The listing builds one solid part. Answer for the finished solid, in the listing's coordinates (mm). Face numbers are marked on the shaded views. A direction names the side the tool comes from. Round coordinates to 2 decimals unless told otherwise and drop trailing zeros. Order: outer loops, then holes, each group sorted by start corner. A loop starts at its lowest first (then second) coordinate and runs counter-clockwise, first axis right, second up. Notation, with made-up numbers: (-38, -1.5) -> (17, -1.5) arc R26 cw to (17, 21.5) -> close; hole circle Ø1 at (-0.5, -27). An arc over 180 degrees is marked (long way). Return JSON: item names as keys, results as strings. Group by question number.
(1) The part is cut by section B-B (x = 23.9). Determine the outline of the cut face in (y, z).
(2) The part is cut by section A-A (z = 18.5). Determine the outline of the cut face in (x, y), plus the area to 3 significant figures.
(3) Consider line 1 (Y direction, x = 0, z = 5.25); line 2 (X direction, y = -35, z = 2.75); line 3 (Y direction, x = 8, z = 14). Determine where each line is inside the solid, lowest interval first. Write a range as [from, to].
(4) The part is cut by section C-C (y = 42.5). Determine the outline of the cut face in (x, z), plus the area to 3 significant figures.
(5) Which of the six approach directions +Z, -Z, +X, -X, +Y, -Y give full straight-line access (tool end or side, diameter ignored) to the marked faces 1, 2, 3, 4 and 5?
(6) The part is cut by section D-D (x = 0). Count the separate pieces of the cut face and the enclosed holes in it, plus the area to 3 significant figures.
(7) Each of these flat-tipped pins is pushed along its axis until it touches: pin 1 (1.1 mm diameter, centred on x = -37.5, y = -14.5, fed in from -Z); pin 2 (2.5 mm diameter, centred on x = 37.5, z = 10, fed in from +Y); pin 3 (4 mm diameter, centred on y = -24, z = 7.5, fed in from +X); pin 4 (2 mm diameter, centred on x = -37, y = 13.5, fed in from +Z). Where does it stop, or does it pass through?
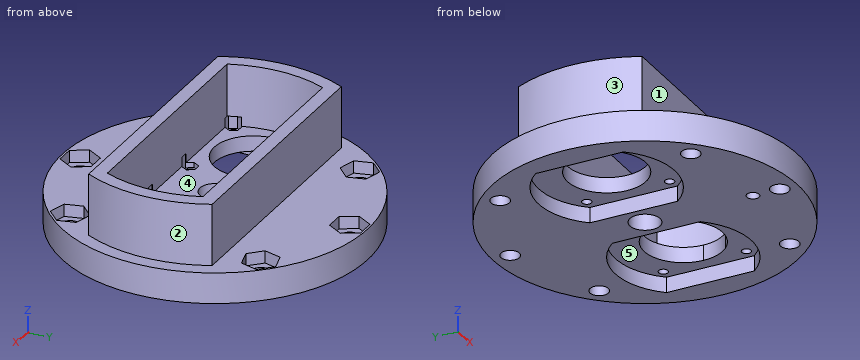
from build123d import *

# Parameters (mm, degrees)
SKETCH2_R               = 49.5
BOSS_EXTRUDE1_DEPTH     = 10
SKETCH1_R               = 1.5
SKETCH1_R_2             = 12.7
CUT_EXTRUDE1_DEPTH      = 5
SKETCH1_12_R            = 4.9
SKETCH1_12_R_2          = 2
CUT_EXTRUDE2_DEPTH      = 45
SKETCH1_13_R            = 1.5
CUT_EXTRUDE3_DEPTH      = 10
BOSS_EXTRUDE2_DEPTH     = 20
SKETCH5_R               = 3
CUT_EXTRUDE4_DEPTH      = 20
SKETCH6_R               = 3
CUT_EXTRUDE5_DEPTH      = 4
CUT_EXTRUDE6_DEPTH      = 3
CUT_EXTRUDE6_DEPTH_BACK = 1.65


with BuildPart() as part:
    # Sketch2 → Boss-Extrude1 (new body)
    with BuildSketch(Plane.XY):
        Circle(SKETCH2_R)
    extrude(amount=BOSS_EXTRUDE1_DEPTH)

    # Sketch1 → Cut-Extrude1 (cut)
    # profile 1 of 2: a face of its own
    with BuildSketch(Plane(origin=(0, 0, 0), x_dir=(-1, 0, 0), z_dir=(0, 0, 1))):
        with BuildLine():
            Line((-7, 14.240786495), (-7, -14.240786495))
            ThreePointArc((-7, -14.240786495), (-23.9, -22.1), (-40.8, -14.240786495))
            Line((-40.8, -14.240786495), (-40.8, 14.240786495))
            ThreePointArc((-40.8, 14.240786495), (-23.9, 22.1), (-7, 14.240786495))
        make_face()
        with Locations(Location((-37.370384182, 13.470384182, 0), (0, 0, 180))):
            Circle(SKETCH1_R, mode=Mode.SUBTRACT)
        with Locations(Location((-10.464971157, 13.435028843, 0), (0, 0, 180))):
            Circle(SKETCH1_R, mode=Mode.SUBTRACT)
        with Locations(Location((-10.464971157, -13.435028843, 0), (0, 0, 180))):
            Circle(SKETCH1_R, mode=Mode.SUBTRACT)
        with Locations(Location((-37.370384182, -13.470384182, 0), (0, 0, 180))):
            Circle(SKETCH1_R, mode=Mode.SUBTRACT)
        with Locations(Location((-23.9, 0, 0), (0, 0, 180))):
            Circle(SKETCH1_R_2, mode=Mode.SUBTRACT)
    # profile 2 of 2: a face of its own
    with BuildSketch(Plane(origin=(0, 0, 0), x_dir=(-1, 0, 0), z_dir=(0, 0, 1))):
        with BuildLine():
            Line((7, 14.240786495), (7, -14.240786495))
            ThreePointArc((7, -14.240786495), (23.9, -22.1), (40.8, -14.240786495))
            Line((40.8, -14.240786495), (40.8, 14.240786495))
            ThreePointArc((40.8, 14.240786495), (23.9, 22.1), (7, 14.240786495))
        make_face()
        with Locations(Location((10.464971157, 13.435028843, 0), (0, 0, 180))):
            Circle(SKETCH1_R, mode=Mode.SUBTRACT)
        with Locations(Location((10.464971157, -13.435028843, 0), (0, 0, 180))):
            Circle(SKETCH1_R, mode=Mode.SUBTRACT)
        with Locations(Location((37.370384182, -13.470384182, 0), (0, 0, 180))):
            Circle(SKETCH1_R, mode=Mode.SUBTRACT)
        with Locations(Location((37.370384182, 13.470384182, 0), (0, 0, 180))):
            Circle(SKETCH1_R, mode=Mode.SUBTRACT)
        with Locations(Location((23.9, 0, 0), (0, 0, 180))):
            Circle(SKETCH1_R_2, mode=Mode.SUBTRACT)
    extrude(amount=CUT_EXTRUDE1_DEPTH, mode=Mode.SUBTRACT)

    # Sketch1<12> → Cut-Extrude2 (cut)
    with BuildSketch(Plane(origin=(0, 0, 0), x_dir=(-1, 0, 0), z_dir=(0, 0, 1))):
        Circle(SKETCH1_12_R)
        with Locations((0, 35)):
            Circle(SKETCH1_12_R_2)
        with BuildLine():
            Line((-11.2, 0), (-23.9, 0))
            Line((-23.9, 0), (-36.6, 0))
            ThreePointArc((-36.6, 0), (-23.9, -12.7), (-11.2, 0))
        make_face()
        with BuildLine():
            Line((-14.919743879, 8.980256121), (-23.9, 0))
            Line((-23.9, 0), (-11.2, 0))
            ThreePointArc((-11.2, 0), (-12.166729937, 4.860079591), (-14.919743879, 8.980256121))
        make_face()
        with BuildLine():
            Line((-32.880256121, 8.980256121), (-23.9, 0))
            Line((-23.9, 0), (-14.919743879, 8.980256121))
            ThreePointArc((-14.919743879, 8.980256121), (-23.9, 12.7), (-32.880256121, 8.980256121))
        make_face()
        with BuildLine():
            Line((-36.6, 0), (-23.9, 0))
            Line((-23.9, 0), (-32.880256121, 8.980256121))
            ThreePointArc((-32.880256121, 8.980256121), (-35.633270063, 4.860079591), (-36.6, 0))
        make_face()
        with BuildLine():
            Line((11.2, 0), (23.9, 0))
            Line((23.9, 0), (36.6, 0))
            ThreePointArc((36.6, 0), (23.9, 12.7), (11.2, 0))
        make_face()
        with BuildLine():
            Line((36.6, 0), (23.9, 0))
            Line((23.9, 0), (11.2, 0))
            ThreePointArc((11.2, 0), (23.9, -12.7), (36.6, 0))
        make_face()
    extrude(amount=CUT_EXTRUDE2_DEPTH, mode=Mode.SUBTRACT)

    # Sketch1<13> → Cut-Extrude3 (cut)
    with BuildSketch(Plane(origin=(0, 0, 0), x_dir=(-1, 0, 0), z_dir=(0, 0, 1))):
        with Locations(Location((-37.370384182, 13.470384182, 0), (0, 0, 180))):
            Circle(SKETCH1_13_R)
        with Locations(Location((-10.464971157, 13.435028843, 0), (0, 0, 180))):
            Circle(SKETCH1_13_R)
        with Locations(Location((-10.464971157, -13.435028843, 0), (0, 0, 180))):
            Circle(SKETCH1_13_R)
        with Locations(Location((-37.370384182, -13.470384182, 0), (0, 0, 180))):
            Circle(SKETCH1_13_R)
        with Locations(Location((10.464971157, 13.435028843, 0), (0, 0, 180))):
            Circle(SKETCH1_13_R)
        with Locations(Location((10.464971157, -13.435028843, 0), (0, 0, 180))):
            Circle(SKETCH1_13_R)
        with Locations(Location((37.370384182, -13.470384182, 0), (0, 0, 180))):
            Circle(SKETCH1_13_R)
        with Locations(Location((37.370384182, 13.470384182, 0), (0, 0, 180))):
            Circle(SKETCH1_13_R)
    extrude(amount=CUT_EXTRUDE3_DEPTH, mode=Mode.SUBTRACT)

    # Sketch4 → Boss-Extrude2 (add)
    with BuildSketch(Plane.XY.offset(10)):
        with BuildLine():
            Line((-40.311288741, -20), (40.311288741, -20))
            ThreePointArc((40.311288741, -20), (45, 0), (40.311288741, 20))
            Line((40.311288741, 20), (-40.311288741, 20))
            ThreePointArc((-40.311288741, 20), (-45, 0), (-40.311288741, -20))
        make_face()
        with BuildLine():
            Line((37.416573868, -15.5), (-37.416573868, -15.5))
            ThreePointArc((-37.416573868, -15.5), (-40.5, 0), (-37.416573868, 15.5))
            Line((-37.416573868, 15.5), (37.416573868, 15.5))
            ThreePointArc((37.416573868, 15.5), (40.5, 0), (37.416573868, -15.5))
        make_face(mode=Mode.SUBTRACT)
    extrude(amount=BOSS_EXTRUDE2_DEPTH)

    # Sketch5 → Cut-Extrude4 (cut)
    with BuildSketch(Plane.XY.offset(10)):
        with Locations((0, 43.7)):
            Circle(SKETCH5_R)
        with Locations((30.900566338, 30.900566338)):
            Circle(SKETCH5_R)
        with Locations((30.900566338, -30.900566338)):
            Circle(SKETCH5_R)
        with Locations((0, -43.7)):
            Circle(SKETCH5_R)
        with Locations((-30.900566338, -30.900566338)):
            Circle(SKETCH5_R)
        with Locations((-30.900566338, 30.900566338)):
            Circle(SKETCH5_R)
    extrude(amount=-CUT_EXTRUDE4_DEPTH, mode=Mode.SUBTRACT)

    # Sketch6 → Cut-Extrude5 (cut)
    # profile 1 of 6: a face of its own
    with BuildSketch(Plane.XY.offset(10)):
        Polygon((-2.915618859, 38.65), (2.915618859, 38.65), (5.831237719, 43.7), (2.915618859, 48.75), (-2.915618859, 48.75), (-5.831237719, 43.7), align=None)
        with Locations((0, 43.7)):
            Circle(SKETCH6_R, mode=Mode.SUBTRACT)
    # profile 2 of 6: a face of its own
    with BuildSketch(Plane.XY.offset(10)):
        Polygon((25.268023226, 29.39133096), (29.39133096, 25.268023226), (35.023874072, 26.777258604), (36.53310945, 32.409801716), (32.409801716, 36.53310945), (26.777258604, 35.023874072), align=None)
        with Locations((30.900566338, 30.900566338)):
            Circle(SKETCH6_R, mode=Mode.SUBTRACT)
    # profile 3 of 6: a face of its own
    with BuildSketch(Plane.XY.offset(10)):
        Polygon((29.39133096, -25.268023226), (25.268023226, -29.39133096), (26.777258604, -35.023874072), (32.409801716, -36.53310945), (36.53310945, -32.409801716), (35.023874072, -26.777258604), align=None)
        with Locations((30.900566338, -30.900566338)):
            Circle(SKETCH6_R, mode=Mode.SUBTRACT)
    # profile 4 of 6: a face of its own
    with BuildSketch(Plane.XY.offset(10)):
        Polygon((2.915618859, -38.65), (-2.915618859, -38.65), (-5.831237719, -43.7), (-2.915618859, -48.75), (2.915618859, -48.75), (5.831237719, -43.7), align=None)
        with Locations((0, -43.7)):
            Circle(SKETCH6_R, mode=Mode.SUBTRACT)
    # profile 5 of 6: a face of its own
    with BuildSketch(Plane.XY.offset(10)):
        Polygon((-25.268023226, -29.39133096), (-29.39133096, -25.268023226), (-35.023874072, -26.777258604), (-36.53310945, -32.409801716), (-32.409801716, -36.53310945), (-26.777258604, -35.023874072), align=None)
        with Locations((-30.900566338, -30.900566338)):
            Circle(SKETCH6_R, mode=Mode.SUBTRACT)
    # profile 6 of 6: a face of its own
    with BuildSketch(Plane.XY.offset(10)):
        Polygon((-26.777258604, 35.023874072), (-32.409801716, 36.53310945), (-36.53310945, 32.409801716), (-35.023874072, 26.777258604), (-29.39133096, 25.268023226), (-25.268023226, 29.39133096), align=None)
    extrude(amount=-CUT_EXTRUDE5_DEPTH, mode=Mode.SUBTRACT)

    # Sketch7 → Cut-Extrude6 (cut, two sides: drawn at the far end of the back side and taken through both)
    with BuildSketch(Plane.XY.offset(10).offset(-CUT_EXTRUDE6_DEPTH_BACK)):
        Polygon((-34.887778024, 13.470384182), (-36.129081103, 15.620384182), (-38.61168726, 15.620384182), (-39.852990339, 13.470384182), (-38.61168726, 11.320384182), (-36.129081103, 11.320384182), align=None)
        Polygon((-9.18831274, -11.320384182), (-11.670918897, -11.320384182), (-12.912221976, -13.470384182), (-11.670918897, -15.620384182), (-9.18831274, -15.620384182), (-7.947009661, -13.470384182), align=None)
        Polygon((-36.129081103, -11.320384182), (-34.887778024, -13.470384182), (-36.129081103, -15.620384182), (-38.61168726, -15.620384182), (-39.852990339, -13.470384182), (-38.61168726, -11.320384182), align=None)
        Polygon((36.129081103, 11.320384182), (34.887778024, 13.470384182), (36.129081103, 15.620384182), (38.61168726, 15.620384182), (39.852990339, 13.470384182), (38.61168726, 11.320384182), align=None)
        Polygon((9.18831274, 11.320384182), (11.670918897, 11.320384182), (12.912221976, 13.470384182), (11.670918897, 15.620384182), (9.18831274, 15.620384182), (7.947009661, 13.470384182), align=None)
        Polygon((7.947009661, -13.470384182), (9.18831274, -11.320384182), (11.670918897, -11.320384182), (12.912221976, -13.470384182), (11.670918897, -15.620384182), (9.18831274, -15.620384182), align=None)
        Polygon((38.61168726, -11.320384182), (36.129081103, -11.320384182), (34.887778024, -13.470384182), (36.129081103, -15.620384182), (38.61168726, -15.620384182), (39.852990339, -13.470384182), align=None)
    extrude(amount=CUT_EXTRUDE6_DEPTH + CUT_EXTRUDE6_DEPTH_BACK, mode=Mode.SUBTRACT)


solid = part.part
Answer below:
{
 "1": {"outline": "(-43.35, 0) -> (-22.1, 0) -> (-22.1, 5) -> (-12.7, 5) -> (-12.7, 10) -> (-15.5, 10) -> (-15.5, 30) -> (-20, 30) -> (-20, 10) -> (-43.35, 10) -> close; (12.7, 5) -> (22.1, 5) -> (22.1, 0) -> (43.35, 0) -> (43.35, 10) -> (20, 10) -> (20, 30) -> (15.5, 30) -> (15.5, 10) -> (12.7, 10) -> close"},
 "2": {"outline": "(-40.31, -20) -> (40.31, -20) arc R45 ccw to (40.31, 20) -> (-40.31, 20) arc R45 ccw to start; hole (-37.42, -15.5) -> (37.42, -15.5) arc R40.5 ccw to (37.42, 15.5) -> (-37.42, 15.5) arc R40.5 ccw to start", "area": "1,030 mm²"},
 "3": {"line 1": "y = [-49.5, -46.7], [-40.7, -37], [-33, -4.9], [4.9, 40.7], [46.7, 49.5]", "line 2": "x = [-35, -2], [2, 35]", "line 3": "y = [-20, -15.5], [15.5, 20]"},
 "4": {"outline": "(-25.38, 0) -> (-2.75, 0) -> (-2.75, 6) -> (-5.14, 6) -> (-5.14, 10) -> (-25.38, 10) -> close; (2.75, 0) -> (25.38, 0) -> (25.38, 10) -> (5.14, 10) -> (5.14, 6) -> (2.75, 6) -> close", "area": "433 mm²"},
 "5": {"face 1": "+Z, +X, -X, -Y", "face 2": "+Z, +X", "face 3": "+Z, -X", "face 4": "+Z", "face 5": "-Z"},
 "6": {"separate pieces": "5", "enclosed holes": "0", "area": "879 mm²"},
 "7": {"pin 1": "stops at z = 5", "pin 2": "stops at y = 33.71", "pin 3": "stops at x = 44.34", "pin 4": "passes through"}
}
